from build123d import *

# Parameters (mm, degrees)
ESQUISSE1_R        = 1.65
ESQUISSE1_R_2      = 6
ESQUISSE1_R_3      = 2.5
ESQUISSE1_W        = 19.5
ESQUISSE1_H        = 27
ESQUISSE1_W_2      = 19
ESQUISSE1_H_2      = 14
BOSS_EXTRU_1_DEPTH = 6


with BuildPart() as part:
    # Esquisse1 → Boss.-Extru.1 (new body)
    with BuildSketch(Plane.XY.offset(-2)):
        Polygon((2459.723805414, -65.693190997), (2443.723805414, -65.693190997), (2443.723805414, -59.693190997), (2423.723805414, -59.693190997), (2423.723805414, -65.693190997), (2393.723805414, -65.693190997), (2393.723805414, -59.693190997), (2373.723805414, -59.693190997), (2373.723805414, -65.693190997), (2351.723805414, -65.693190997), (2351.723805414, -25.693190997), (2357.723805414, -25.693190997), (2357.723805414, 14.306809003), (2351.723805414, 14.306809003), (2351.723805414, 54.306809003), (2357.723805414, 54.306809003), (2357.723805414, 94.306809003), (2351.723805414, 94.306809003), (2351.723805414, 134.306809003), (2357.723805414, 134.306809003), (2357.723805414, 181.409908735), (2373.723805414, 181.409908735), (2373.723805414, 175.409908735), (2393.723805414, 175.409908735), (2393.723805414, 181.409908735), (2423.723805414, 181.409908735), (2423.723805414, 175.409908735), (2443.723805414, 175.409908735), (2443.723805414, 181.409908735), (2453.723805414, 181.409908735), (2453.723805414, 134.306809003), (2459.723805414, 134.306809003), (2459.723805414, 94.306809003), (2453.723805414, 94.306809003), (2453.723805414, 54.306809003), (2459.723805414, 54.306809003), (2459.723805414, 14.306809003), (2453.723805414, 14.306809003), (2453.723805414, -25.693190997), (2459.723805414, -25.693190997), align=None)
        with Locations((2411.223763127, 102.806809003)):
            Circle(ESQUISSE1_R, mode=Mode.SUBTRACT)
        with Locations((2419.723805414, 94.306851291)):
            Circle(ESQUISSE1_R, mode=Mode.SUBTRACT)
        with Locations((2411.223805414, 94.306809003)):
            Circle(ESQUISSE1_R_2, mode=Mode.SUBTRACT)
        with Locations((2402.723805414, 94.306766716)):
            Circle(ESQUISSE1_R, mode=Mode.SUBTRACT)
        with Locations((2411.223847701, 85.806809003)):
            Circle(ESQUISSE1_R, mode=Mode.SUBTRACT)
        with Locations((2442.573805414, 102.010809003)):
            Circle(ESQUISSE1_R_3, mode=Mode.SUBTRACT)
        with Locations((2379.523805414, 61.806809003)):
            Rectangle(ESQUISSE1_W, ESQUISSE1_H, mode=Mode.SUBTRACT)
        with BuildLine():
            Line((2366.723805414, 71.506809003), (2366.723805414, 72.706809003))
            ThreePointArc((2366.723805414, 72.706809003), (2367.873805414, 73.856809003), (2369.023805414, 72.706809003))
            Line((2369.023805414, 72.706809003), (2369.023805414, 71.506809003))
            ThreePointArc((2369.023805414, 71.506809003), (2367.873805414, 70.356809003), (2366.723805414, 71.506809003))
        make_face(mode=Mode.SUBTRACT)
        with BuildLine():
            Line((2392.323805414, 72.706809003), (2392.323805414, 71.506809003))
            ThreePointArc((2392.323805414, 71.506809003), (2391.173805414, 70.356809003), (2390.023805414, 71.506809003))
            Line((2390.023805414, 71.506809003), (2390.023805414, 72.706809003))
            ThreePointArc((2390.023805414, 72.706809003), (2391.173805414, 73.856809003), (2392.323805414, 72.706809003))
        make_face(mode=Mode.SUBTRACT)
        with BuildLine():
            Line((2392.323805414, 52.106809003), (2392.323805414, 50.906809003))
            ThreePointArc((2392.323805414, 50.906809003), (2391.173805414, 49.756809003), (2390.023805414, 50.906809003))
            Line((2390.023805414, 50.906809003), (2390.023805414, 52.106809003))
            ThreePointArc((2390.023805414, 52.106809003), (2391.173805414, 53.256809003), (2392.323805414, 52.106809003))
        make_face(mode=Mode.SUBTRACT)
        with BuildLine():
            Line((2366.723805414, 52.106809003), (2366.723805414, 50.906809003))
            ThreePointArc((2366.723805414, 50.906809003), (2367.873805414, 49.756809003), (2369.023805414, 50.906809003))
            Line((2369.023805414, 50.906809003), (2369.023805414, 52.106809003))
            ThreePointArc((2369.023805414, 52.106809003), (2367.873805414, 53.256809003), (2366.723805414, 52.106809003))
        make_face(mode=Mode.SUBTRACT)
        with BuildLine():
            Line((2418.073805414, -9.193190997), (2418.073805414, -12.193190997))
            ThreePointArc((2418.073805414, -12.193190997), (2419.723805414, -13.843190997), (2421.373805414, -12.193190997))
            Line((2421.373805414, -12.193190997), (2421.373805414, -9.193190997))
            ThreePointArc((2421.373805414, -9.193190997), (2419.723805414, -7.543190997), (2418.073805414, -9.193190997))
        make_face(mode=Mode.SUBTRACT)
        with BuildLine():
            Line((2401.073805414, -9.193190997), (2401.073805414, -12.193190997))
            ThreePointArc((2401.073805414, -12.193190997), (2402.723805414, -13.843190997), (2404.373805414, -12.193190997))
            Line((2404.373805414, -12.193190997), (2404.373805414, -9.193190997))
            ThreePointArc((2404.373805414, -9.193190997), (2402.723805414, -7.543190997), (2401.073805414, -9.193190997))
        make_face(mode=Mode.SUBTRACT)
        with BuildLine():
            Line((2405.223805414, -9.193190997), (2405.223805414, -12.193190997))
            ThreePointArc((2405.223805414, -12.193190997), (2411.223805414, -18.193190997), (2417.223805414, -12.193190997))
            Line((2417.223805414, -12.193190997), (2417.223805414, -9.193190997))
            ThreePointArc((2417.223805414, -9.193190997), (2411.223805414, -3.193190997), (2405.223805414, -9.193190997))
        make_face(mode=Mode.SUBTRACT)
        with Locations((2435.223805414, 80.010809003)):
            Rectangle(ESQUISSE1_W_2, ESQUISSE1_H_2, mode=Mode.SUBTRACT)
        with BuildLine():
            Line((2448.123805414, 68.756809003), (2448.123805414, 62.756809003))
            ThreePointArc((2448.123805414, 62.756809003), (2447.391572367, 60.98904205), (2445.623805414, 60.256809003))
            Line((2445.623805414, 60.256809003), (2437.623805414, 60.256809003))
            ThreePointArc((2437.623805414, 60.256809003), (2435.856038461, 60.98904205), (2435.123805414, 62.756809003))
            Line((2435.123805414, 62.756809003), (2435.123805414, 68.756809003))
            ThreePointArc((2435.123805414, 68.756809003), (2435.856038461, 70.524575956), (2437.623805414, 71.256809003))
            Line((2437.623805414, 71.256809003), (2445.623805414, 71.256809003))
            ThreePointArc((2445.623805414, 71.256809003), (2447.391572367, 70.524575956), (2448.123805414, 68.756809003))
        make_face(mode=Mode.SUBTRACT)
        Polygon((2386.739083665, -41.66500263), (2387.836028015, -31.150640303), (2389.825231698, -31.358170315), (2388.728287348, -41.872532642), align=None, mode=Mode.SUBTRACT)
        Polygon((2388.932972364, -20.636277977), (2390.029916714, -10.12191565), (2392.019120398, -10.329445662), (2390.922176048, -20.843807989), align=None, mode=Mode.SUBTRACT)
        Polygon((2391.126861064, 0.392446677), (2392.223805414, 10.906809003), (2394.213009097, 10.699278991), (2393.116064748, 0.184916664), align=None, mode=Mode.SUBTRACT)
    extrude(amount=BOSS_EXTRU_1_DEPTH)


solid = part.part
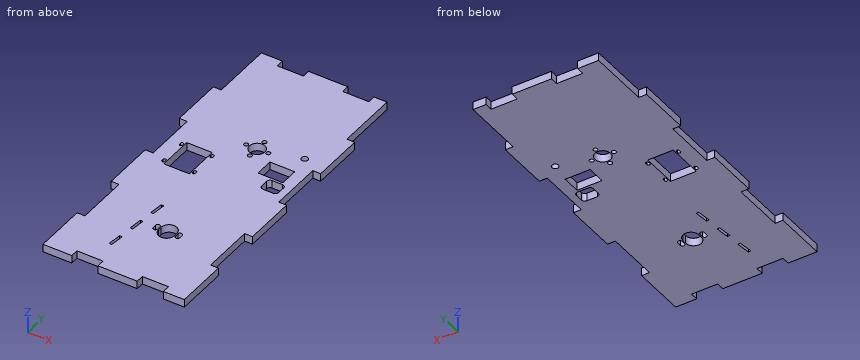
Can you work these out from the model? Positions are in its coordinate system, mm. Coordinates: 2 decimals unless noted, no trailing zeros. Write each loop counter-clockwise with the first axis right and the second up, starting at its lowest first coordinate (ties: lowest second). Pieces come first, ordered by that corner, then holes. Notation, with made-up numbers: (46.5, 77) -> (104.5, 77) arc R9 ccw to (104.5, 89) -> close; hole circle Ø7 at (58.25, 23.5). An arc over 180 degrees is marked (long way). Write each question's results on one line, items separated by ' | '. Start each with the question number.
Item 1: If we section it at A-A, the plane y = 152: Write out the boundary of the cut face in (x, z).
Item 2: If we section it at B-B, the plane z = 1.3: Count the separate pieces of the cut face and the enclosed holes in it, and give its area (3 significant figures).
Item 3: Please list where these lines run through material, in increasing order: probe 1 along X at (y, z) = (94.5, -0.75); probe 2 along Y at (x, z) = (2454, 0); probe 3 along X at (y, z) = (-31.5, 0).
Item 4: I'm going to push flat-ended pins straight in: P1, Ø3, axis at x = 2457.5, z = 0.5, coming from the +Y side; P2, Ø8, axis at x = 2389.5, y = -18, coming from the -Z side; P3, Ø1.8, axis at y = 177.5, z = 0.5, coming from the -X side; P4, Ø0.9, axis at y = -11, z = 0, coming from the +X side. Where does each tip first touch, or does it pass through?
Answer block:
1) outline: (2357.72, -2) -> (2453.72, -2) -> (2453.72, 4) -> (2357.72, 4) -> close
2) separate pieces: 1 | enclosed holes: 19 | area: 23,300 mm²
3) probe 1: 2351.72 to 2401.09, 2404.36 to 2405.23, 2417.22 to 2418.09, 2421.36 to 2459.72 | probe 2: -65.69 to -25.69, 14.31 to 54.31, 94.31 to 134.31 | probe 3: 2351.72 to 2387.8, 2389.81 to 2459.72
4) P1: y = 134.31 | P2: z = -2 | P3: x = 2357.72 | P4: x = 2453.72
